from build123d import *

# Parameters (mm, degrees)
SKETCH1_W            = 6.35
SKETCH1_H            = 5.842
BOSS_EXTRUDE1_DEPTH  = 3.175
BOSS_EXTRUDE2_DEPTH  = 5.08
SKETCH3_W            = 5.842
SKETCH3_H            = 3.175
BOSS_EXTRUDE3_DEPTH  = 1.27
SKETCH4_W            = 1.651
SKETCH4_H            = 0.635
CUT_EXTRUDE1_DEPTH   = 6.842
SKETCH5_W            = 0.635
SKETCH5_H            = 0.635
BOSS_EXTRUDE4_DEPTH  = 3.6725
SKETCH6_W            = 0.635
SKETCH6_H            = 0.635
BOSS_EXTRUDE5_DEPTH  = 6.4543
SKETCH7_W            = 1.651
SKETCH7_H            = 0.635
CUT_EXTRUDE2_DEPTH   = 10.642
SKETCH8_W            = 0.635
SKETCH8_H            = 0.635
BOSS_EXTRUDE6_DEPTH  = 3.6725
SKETCH9_W            = 0.635
SKETCH9_H            = 0.635
BOSS_EXTRUDE7_DEPTH  = 6.4543
SKETCH10_W           = 1.651
SKETCH10_H           = 0.635
CUT_EXTRUDE3_DEPTH   = 10.642
SKETCH11_W           = 0.635
SKETCH11_H           = 0.635
BOSS_EXTRUDE8_DEPTH  = 3.6725
SKETCH12_W           = 0.635
SKETCH12_H           = 0.635
BOSS_EXTRUDE9_DEPTH  = 6.4543
SKETCH13_W           = 0.635
SKETCH13_H           = 0.635
BOSS_EXTRUDE10_DEPTH = 6.71
SKETCH14_W           = 0.635
SKETCH14_H           = 0.635
BOSS_EXTRUDE11_DEPTH = 6.71
SKETCH15_W           = 0.635
SKETCH15_H           = 0.635
BOSS_EXTRUDE12_DEPTH = 6.71
SKETCH16_W           = 0.635
SKETCH16_H           = 1.27
CUT_EXTRUDE4_DEPTH   = 1.27
SKETCH17_W           = 0.635
SKETCH17_H           = 1.27
CUT_EXTRUDE5_DEPTH   = 1.27
CHAMFER1_SIZE        = 0.127
CHAMFER2_SIZE        = 0.753913762
CHAMFER2_SIZE2       = 0.55706549
FILLET1_R            = 1
FILLET2_R            = 1.635


with BuildPart() as part:
    # Sketch1 → Boss-Extrude1 (new body)
    with BuildSketch(Plane.XZ.offset(1.5875)):
        with Locations((-0.635, 0.0508)):
            Rectangle(SKETCH1_W, SKETCH1_H)
    extrude(amount=-BOSS_EXTRUDE1_DEPTH)

    # Sketch2 → Boss-Extrude2 (add)
    with BuildSketch(Plane(origin=(2.54, 0, 0), x_dir=(0, 0, -1), z_dir=(1, 0, 0))):
        Polygon((0.651, 4.6355), (1.8702, 3.4925), (1.8702, 1.5875), (2.8702, 1.5875), (2.8702, 10.1125), (1.8702, 10.1125), (1.8702, 6.5405), align=None)
    extrude(amount=-BOSS_EXTRUDE2_DEPTH)

    # Sketch3 → Boss-Extrude3 (add)
    with BuildSketch(Plane(origin=(2.54, 0, 0), x_dir=(0, 0, -1), z_dir=(1, 0, 0))):
        with Locations((-0.0508, 0)):
            Rectangle(SKETCH3_W, SKETCH3_H)
    extrude(amount=BOSS_EXTRUDE3_DEPTH)

    # Sketch4 → Cut-Extrude1 (cut, through all)
    with BuildSketch(Plane(origin=(0, 0, -2.8702), x_dir=(-1, 0, 0), z_dir=(0, 0, -1))):
        with Locations((0, -1.27)):
            Rectangle(SKETCH4_W, SKETCH4_H)
    extrude(amount=-CUT_EXTRUDE1_DEPTH, mode=Mode.SUBTRACT)

    # Sketch5 → Boss-Extrude4 (add)
    with BuildSketch(Plane.XZ.offset(0.9525)):
        Rectangle(SKETCH5_W, SKETCH5_H)
    extrude(amount=BOSS_EXTRUDE4_DEPTH)

    # Sketch6 → Boss-Extrude5 (add)
    with BuildSketch(Plane.XY.offset(0.3175)):
        with Locations((0, -4.3075)):
            Rectangle(SKETCH6_W, SKETCH6_H)
    extrude(amount=BOSS_EXTRUDE5_DEPTH)

    # Sketch7 → Cut-Extrude2 (cut, through all)
    with BuildSketch(Plane(origin=(0, 0, -2.8702), x_dir=(-1, 0, 0), z_dir=(0, 0, -1))):
        with Locations((2.54, -1.27)):
            Rectangle(SKETCH7_W, SKETCH7_H)
    extrude(amount=-CUT_EXTRUDE2_DEPTH, mode=Mode.SUBTRACT)

    # Sketch8 → Boss-Extrude6 (add)
    with BuildSketch(Plane.XZ.offset(0.9525)):
        with Locations((-2.54, 0)):
            Rectangle(SKETCH8_W, SKETCH8_H)
    extrude(amount=BOSS_EXTRUDE6_DEPTH)

    # Sketch9 → Boss-Extrude7 (add)
    with BuildSketch(Plane.XY.offset(0.3175)):
        with Locations((-2.54, -4.3075)):
            Rectangle(SKETCH9_W, SKETCH9_H)
    extrude(amount=BOSS_EXTRUDE7_DEPTH)

    # Sketch10 → Cut-Extrude3 (cut, through all)
    with BuildSketch(Plane(origin=(0, 0, -2.8702), x_dir=(-1, 0, 0), z_dir=(0, 0, -1))):
        with Locations((-2.54, -1.27)):
            Rectangle(SKETCH10_W, SKETCH10_H)
    extrude(amount=-CUT_EXTRUDE3_DEPTH, mode=Mode.SUBTRACT)

    # Sketch11 → Boss-Extrude8 (add)
    with BuildSketch(Plane.XZ.offset(0.9525)):
        with Locations((2.54, 0)):
            Rectangle(SKETCH11_W, SKETCH11_H)
    extrude(amount=BOSS_EXTRUDE8_DEPTH)

    # Sketch12 → Boss-Extrude9 (add)
    with BuildSketch(Plane.XY.offset(0.3175)):
        with Locations((2.54, -4.3075)):
            Rectangle(SKETCH12_W, SKETCH12_H)
    extrude(amount=BOSS_EXTRUDE9_DEPTH)

    # Sketch13 → Boss-Extrude10 (add)
    with BuildSketch(Plane(origin=(0, 1.5875, 0), x_dir=(-1, 0, 0), z_dir=(0, 1, 0))):
        with Locations((-2.54, 0)):
            Rectangle(SKETCH13_W, SKETCH13_H)
    extrude(amount=BOSS_EXTRUDE10_DEPTH)

    # Sketch14 → Boss-Extrude11 (add)
    with BuildSketch(Plane(origin=(0, 1.5875, 0), x_dir=(-1, 0, 0), z_dir=(0, 1, 0))):
        Rectangle(SKETCH14_W, SKETCH14_H)
    extrude(amount=BOSS_EXTRUDE11_DEPTH)

    # Sketch15 → Boss-Extrude12 (add)
    with BuildSketch(Plane(origin=(0, 1.5875, 0), x_dir=(-1, 0, 0), z_dir=(0, 1, 0))):
        with Locations((2.54, 0)):
            Rectangle(SKETCH15_W, SKETCH15_H)
    extrude(amount=BOSS_EXTRUDE12_DEPTH)

    # Sketch16 → Cut-Extrude4 (cut)
    with BuildSketch(Plane(origin=(0, 1.5875, 0), x_dir=(-1, 0, 0), z_dir=(0, 1, 0))):
        with Locations((-1.27, 0)):
            Rectangle(SKETCH16_W, SKETCH16_H)
    extrude(amount=-CUT_EXTRUDE4_DEPTH, mode=Mode.SUBTRACT)

    # Sketch17 → Cut-Extrude5 (cut)
    with BuildSketch(Plane(origin=(0, 1.5875, 0), x_dir=(-1, 0, 0), z_dir=(0, 1, 0))):
        with Locations((1.27, 0)):
            Rectangle(SKETCH17_W, SKETCH17_H)
    extrude(amount=-CUT_EXTRUDE5_DEPTH, mode=Mode.SUBTRACT)

    # Chamfer1
    chamfer1_edges = [part.edges().sort_by_distance(p)[0] for p in [
        (-2.54, -3.99, 6.7718),
        (-2.8575, -4.3075, 6.7718),
        (-2.54, -4.625, 6.7718),
        (-2.2225, -4.3075, 6.7718),
        (2.8575, -4.3075, 6.7718),
        (2.54, -3.99, 6.7718),
        (2.2225, -4.3075, 6.7718),
        (2.54, -4.625, 6.7718),
        (2.2225, 8.2975, 0),
        (2.54, 8.2975, 0.3175),
        (2.8575, 8.2975, 0),
        (2.54, 8.2975, -0.3175),
        (0.3175, 8.2975, 0),
        (0, 8.2975, -0.3175),
        (-0.3175, 8.2975, 0),
        (0, 8.2975, 0.3175),
        (-2.54, 8.2975, 0.3175),
        (-2.2225, 8.2975, 0),
        (-2.54, 8.2975, -0.3175),
        (-2.8575, 8.2975, 0),
        (0, -3.99, 6.7718),
        (-0.3175, -4.3075, 6.7718),
        (0, -4.625, 6.7718),
        (0.3175, -4.3075, 6.7718),
    ]]
    chamfer(chamfer1_edges, length=CHAMFER1_SIZE)

    # Chamfer2
    chamfer2_edges = [part.edges().sort_by_distance(p)[0] for p in [
        (0, 4.6355, -0.651),
    ]]
    chamfer2_side = [part.faces().sort_by_distance(p)[0] for p in [
        (0, 5.588, -1.2606),
    ]]
    chamfer(chamfer2_edges, length=CHAMFER2_SIZE, length2=CHAMFER2_SIZE2, reference=chamfer2_side[0])

    # Fillet1
    fillet1_edges = [part.edges().sort_by_distance(p)[0] for p in [
        (-2.54, -3.99, 0.3175),
        (2.54, -3.99, 0.3175),
        (0, -3.99, 0.3175),
    ]]
    fillet(fillet1_edges, radius=FILLET1_R)

    # Fillet2
    fillet2_edges = [part.edges().sort_by_distance(p)[0] for p in [
        (-2.54, -4.625, -0.3175),
        (2.54, -4.625, -0.3175),
        (0, -4.625, -0.3175),
    ]]
    fillet(fillet2_edges, radius=FILLET2_R)


solid = part.part
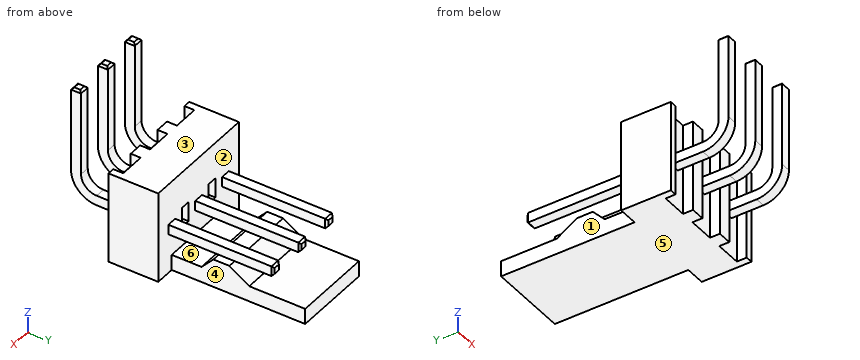
Geometry check sheet. Reference: the model listing, model coordinates, mm. Face numbers are marked on the shaded views. A direction names the side the tool comes from. Round coordinates to 2 decimals unless told otherwise and drop trailing zeros. Loops run counter-clockwise (first coordinate to the right, second up) from the corner with the lowest first, then second, coordinate; pieces in that order, holes last.
Item 1: Thickness scan on line 1 (X direction, y = 6, z = 0.25); line 2 (Y direction, x = 3, z = -0.25); line 3 (Y direction, x = 2.5, z = 6) (3 decimals). Record the ranges inside material, lowest first.
Item 2: Cross-section at A-A on y = 3. Record the boundary of the cut face in (x, z), then the cut area to 3 significant figures.
Item 3: Cross-section at C-C on z = 1. Record the boundary of the cut face in (x, y), then the cut area to 3 significant figures.
Item 4: Access from +Z, -Z, +X, -X, +Y, -Y to the whole of each face (thin tool, end or side, straight path). Record for the marked faces 3, 4, 5 and 6.
Item 5: Cross-section at D-D on x = -0.5. Record the boundary of the cut face in (y, z), then the cut area to 3 significant figures.
Item 6: Cross-section at B-B on y = 1.25. Record the boundary of the cut face in (x, z) (1 decimal), then the cut area to 3 significant figures.
Item 7: Mould release check, pull along Y, two halves, no side actions. Record for the marked faces 1 and 2: pulls with the +Y half, pulls with the -Y half, needs draft (parallel to the pull), parting line crosses it, or undercut.
Item 8: Gauge pin test, flat ends, axial feed: pin 1 (1.8 mm diameter, centred on y = -3, z = 3, fed in from -X); pin 2 (4 mm diameter, centred on y = -3, z = 3.5, fed in from +X); pin 3 (0.7 mm diameter, centred on x = -1.5, y = 1, fed in from +Z); pin 4 (0.5 mm diameter, centred on x = 2.5, y = 3.5, fed in from +Z). Record the tip position at first contact, or that the pin passes through.
Answer sheet:
1. line 1: x = -2.86 to -2.22, -0.32 to 0.32, 2.22 to 2.86
1. line 2: y = -0.95 to 1.59
1. line 3: y = -4.625 to -3.99
2. outline: (-2.86, -0.32) - (-2.22, -0.32) - (-2.22, 0.32) - (-2.86, 0.32) - close; (-2.54, -2.87) - (2.54, -2.87) - (2.54, -1.87) - (-2.54, -1.87) - close; (-0.32, -0.32) - (0.32, -0.32) - (0.32, 0.32) - (-0.32, 0.32) - close; (2.22, -0.32) - (2.86, -0.32) - (2.86, 0.32) - (2.22, 0.32) - close
2. area: 6.29 mm2
3. outline: (-3.81, -1.59) - (-3.37, -1.59) - (-3.37, -0.95) - (-1.71, -0.95) - (-1.71, -1.59) - (-0.83, -1.59) - (-0.83, -0.95) - (0.83, -0.95) - (0.83, -1.59) - (1.71, -1.59) - (1.71, -0.95) - (3.37, -0.95) - (3.37, -1.59) - (3.81, -1.59) - (3.81, 1.59) - (-3.81, 1.59) - close; (-2.86, -4.59) - (-2.22, -4.59) - (-2.22, -3.94) - (-2.86, -3.94) - close; (-0.32, -4.59) - (0.32, -4.59) - (0.32, -3.94) - (-0.32, -3.94) - close; (2.22, -4.59) - (2.86, -4.59) - (2.86, -3.94) - (2.22, -3.94) - close
3. area: 22.3 mm2
4. face 3: +Z, +X, -X, +Y
4. face 4: -Z, +X, +Y
4. face 5: -Z, +X, -X, +Y, -Y
4. face 6: +X, -X
5. outline: (-0.95, -2.87) - (10.11, -2.87) - (10.11, -1.87) - (6.54, -1.87) - (5.27, -1.06) - (4.25, -1.06) - (3.49, -1.87) - (1.59, -1.87) - (1.59, 2.97) - (-0.95, 2.97) - close
5. area: 25.0 mm2
6. outline: (-3.8, -2.9) - (3.8, -2.9) - (3.8, 3) - (-3.8, 3) - close; hole (-1.6, -0.6) - (-1, -0.6) - (-1, 0.6) - (-1.6, 0.6) - close; hole (1, -0.6) - (1.6, -0.6) - (1.6, 0.6) - (1, 0.6) - close
6. area: 42.9 mm2
7. face 1: needs draft
7. face 2: undercut
8. pin 1: passes through
8. pin 2: stops at x = 3.81
8. pin 3: stops at z = 2.97
8. pin 4: stops at z = 0.32
